Input: part model. Units: mm. Frame: model coordinates. A direction names the side the tool comes from. Round coordinates to 2 decimals unless told otherwise and drop trailing zeros. Use a Markdown table: item, result.
from build123d import *

# Parameters (mm, degrees)
BR_EXTRUDE_DEPTH      = 110
BR_EXTRUDE_DEPTH_BACK = 110


with BuildPart() as part:
    # Sketch2 → BR_Extrude (new, two sides: drawn at the far end of the back side and taken through both)
    with BuildSketch(Plane(origin=(0, 0, 0), x_dir=(0, 0, -1), z_dir=(1, 0, 0)).offset(-BR_EXTRUDE_DEPTH_BACK)):
        with BuildLine():
            Line((-7.060660172, -6), (-8.5, -6))
            Line((-8.5, -6), (-8.5, -3))
            Line((-8.5, -3), (-9.5, -3))
            Line((-9.5, -3), (-9.5, -3.5))
            Line((-9.5, -3.5), (-10, -3.5))
            Line((-10, -3.5), (-10, -8.5))
            ThreePointArc((-10, -8.5), (-9.560660172, -9.560660172), (-8.5, -10))
            Line((-8.5, -10), (-3.5, -10))
            Line((-3.5, -10), (-3.5, -9.5))
            Line((-3.5, -9.5), (-3, -9.5))
            Line((-3, -9.5), (-3, -8.5))
            Line((-3, -8.5), (-6, -8.5))
            Line((-6, -8.5), (-6, -7.060660172))
            Line((-6, -7.060660172), (-3.439339828, -4.5))
            Line((-3.439339828, -4.5), (3.439339828, -4.5))
            Line((3.439339828, -4.5), (6, -7.060660172))
            Line((6, -7.060660172), (6, -8.5))
            Line((6, -8.5), (3, -8.5))
            Line((3, -8.5), (3, -9.5))
            Line((3, -9.5), (3.5, -9.5))
            Line((3.5, -9.5), (3.5, -10))
            Line((3.5, -10), (8.5, -10))
            ThreePointArc((8.5, -10), (9.560660172, -9.560660172), (10, -8.5))
            Line((10, -8.5), (10, -3.5))
            Line((10, -3.5), (9.5, -3.5))
            Line((9.5, -3.5), (9.5, -3))
            Line((9.5, -3), (8.5, -3))
            Line((8.5, -3), (8.5, -6))
            Line((8.5, -6), (7.060660172, -6))
            Line((7.060660172, -6), (4.5, -3.439339828))
            Line((4.5, -3.439339828), (4.5, 3.439339828))
            Line((4.5, 3.439339828), (7.060660172, 6))
            Line((7.060660172, 6), (8.5, 6))
            Line((8.5, 6), (8.5, 3))
            Line((8.5, 3), (9.5, 3))
            Line((9.5, 3), (9.5, 3.5))
            Line((9.5, 3.5), (10, 3.5))
            Line((10, 3.5), (10, 8.5))
            ThreePointArc((10, 8.5), (9.560660172, 9.560660172), (8.5, 10))
            Line((8.5, 10), (3.5, 10))
            Line((3.5, 10), (3.5, 9.5))
            Line((3.5, 9.5), (3, 9.5))
            Line((3, 9.5), (3, 8.5))
            Line((3, 8.5), (6, 8.5))
            Line((6, 8.5), (6, 7.060660172))
            Line((6, 7.060660172), (3.439339828, 4.5))
            Line((3.439339828, 4.5), (-3.439339828, 4.5))
            Line((-3.439339828, 4.5), (-6, 7.060660172))
            Line((-6, 7.060660172), (-6, 8.5))
            Line((-6, 8.5), (-3, 8.5))
            Line((-3, 8.5), (-3, 9.5))
            Line((-3, 9.5), (-3.5, 9.5))
            Line((-3.5, 9.5), (-3.5, 10))
            Line((-3.5, 10), (-8.5, 10))
            ThreePointArc((-8.5, 10), (-9.560660172, 9.560660172), (-10, 8.5))
            Line((-10, 8.5), (-10, 3.5))
            Line((-10, 3.5), (-9.5, 3.5))
            Line((-9.5, 3.5), (-9.5, 3))
            Line((-9.5, 3), (-8.5, 3))
            Line((-8.5, 3), (-8.5, 6))
            Line((-8.5, 6), (-7.060660172, 6))
            Line((-7.060660172, 6), (-4.5, 3.439339828))
            Line((-4.5, 3.439339828), (-4.5, -3.439339828))
            Line((-4.5, -3.439339828), (-7.060660172, -6))
        make_face()
        with BuildLine():
            Line((-3.000174203, -1.949573265), (-2.435636363, -1.276783266))
            ThreePointArc((-2.435636363, -1.276783266), (-2.75, 0), (-2.435636363, 1.276783266))
            Line((-2.435636363, 1.276783266), (-3.000174203, 1.949573265))
            Line((-3.000174203, 1.949573265), (-1.949573265, 3.000174203))
            Line((-1.949573265, 3.000174203), (-1.276783266, 2.435636363))
            ThreePointArc((-1.276783266, 2.435636363), (0, 2.75), (1.276783266, 2.435636363))
            Line((1.276783266, 2.435636363), (1.949573265, 3.000174203))
            Line((1.949573265, 3.000174203), (3.000174203, 1.949573265))
            Line((3.000174203, 1.949573265), (2.435636363, 1.276783266))
            ThreePointArc((2.435636363, 1.276783266), (2.75, 0), (2.435636363, -1.276783266))
            Line((2.435636363, -1.276783266), (3.000174203, -1.949573265))
            Line((3.000174203, -1.949573265), (1.949573265, -3.000174203))
            Line((1.949573265, -3.000174203), (1.276783266, -2.435636363))
            ThreePointArc((1.276783266, -2.435636363), (0, -2.75), (-1.276783266, -2.435636363))
            Line((-1.276783266, -2.435636363), (-1.949573265, -3.000174203))
            Line((-1.949573265, -3.000174203), (-3.000174203, -1.949573265))
        make_face(mode=Mode.SUBTRACT)
    extrude(amount=BR_EXTRUDE_DEPTH + BR_EXTRUDE_DEPTH_BACK)


solid = part.part
1) Contact query for flat-ended pins moving along their axis: P1, Ø2, axis at x = -21, y = -1.5, coming from the -Z side; P2, Ø0.6, axis at x = -49, z = 10, coming from the +Y side; P3, Ø0.6, axis at x = 28.5, y = 3, coming from the +Z side. Output: stop coordinate, or through.
Answer key:
| item | result |
|---|---|
| P1 | stops at z = -4.5 |
| P2 | stops at y = 9.4 |
| P3 | stops at z = 9.5 |
2) Set-up query: faces 4 (the face through (-2, 0, -4.5)), 5 (the face through (-2, 10, 6)). Return all of +Z, -Z, +X, -X, +Y, -Y with unobstructed straight access to the full face (end or side cutting, diameter ignored); none if empty.
Answer key:
| item | result |
|---|---|
| face 4 | +X, -X |
| face 5 | +Z, -Z, +X, -X, +Y |
3) Ray query, probe 1 along Y at (x, z) = (95, 3.25); probe 2 along Z at (x, y) = (-98.5, -7.5); probe 3 along Y at (x, z) = (-91, 1.25). Return the intervals inside material, ascending.
Answer key:
| item | result |
|---|---|
| probe 1 | y = -9.5 to -8.5, -4.5 to 4.5, 8.5 to 9.5 |
| probe 2 | z = -10 to -6, 6 to 10 |
| probe 3 | y = -4.5 to -2.45, 2.45 to 4.5 |
4) Draft query along Y for faces 1 (the face through (-2, -10, -6)), 2 (the face through (110, -4, 0)), 3 (the face through (-2, 0, 4.5)). Return one class per face: released by +Y, released by -Y, zero draft, split by the parting line, or undercut.
Answer key:
| item | result |
|---|---|
| face 1 | released by -Y |
| face 2 | zero draft |
| face 3 | undercut |
